Read the model definition and answer for the solid it produces. Units are mm, in the model's axes. A direction names the side the tool comes from. Round coordinates to 2 decimals unless told otherwise and drop trailing zeros. Loops run counter-clockwise (first coordinate to the right, second up) from the corner with the lowest first, then second, coordinate; pieces in that order, holes last. Notation, with made-up numbers: (31, 23.25) - (62, 23.25) arc R22 cw to (62, 57.25) - close; hole circle Ø7 at (-0.75, -3.75). An arc over 180 degrees is marked (long way). Use CSV: the item, a comma, the result in double quotes. Start each with the question number.
1. Consider line 1 along Y through (x, z) = (1.5, 0); line 2 along Z through (x, y) = (-34.5, -29); line 3 along X through (y, z) = (-25, 4). Determine where each line is inside the solid, lowest interval first.
2. A tool of negligible diameter and unlimited length cuts with its end or side. For faces 1 (the flat face through (1, -12.7, 7)), 2 (the flat face through (-19.164, -18, 5)), 3 (the flat face through (-12.7, -22.4, 9.3)), from which of +Z, -Z, +X, -X, +Y, -Y can it reach the whole face along a straight path? Write none if from no direction.
3. Find section D-D (z = 1.5). Give the vertices of the cut face in (x, y), and give its area (3 significant figures).
4. Given pin 1 Ø5.5 at (x, y) = (-29, -18.5) entering from +Z; pin 2 Ø5.5 at (x, z) = (-1.5, 10.5) entering from -Y; pin 3 Ø15 at (y, z) = (-27, 9) entering from +X, each flat-ended and moving along its own axis, determine where each tip first touches the part or whether it passes through.
5. Find section C-C (x = -9). Give the vertices of the cut face in (y, z).
6. Find section B-B (z = 13.5). Give the vertices of the cut face in (x, y).
7. Find section A-A (y = -8). Give the vertices of the cut face in (x, z), and give its area (3 significant figures).
from build123d import *

# Parameters (mm, degrees)
F0_W      = 50.8
F0_H      = 31.75
F1_DEPTH  = 31.75
F3_DEPTH  = 31.75
F5_DEPTH  = 19.05
F6_W      = 19.05
F6_H      = 18.953177
F7_DEPTH  = 19.05
F9_DEPTH  = 12.7
F11_DEPTH = 25.4


with BuildPart() as f1:
    # F0 (on Front) → F1 (new body)
    with BuildSketch(Plane.XZ):
        with Locations((-12.814426, 3.078177)):
            Rectangle(F0_W, F0_H)
    extrude(amount=F1_DEPTH)

    # F2 (on face) → F3 (cut)
    with BuildSketch(Plane.XZ.offset(31.75)):
        Polygon((12.585574, -0.096823), (12.585574, 18.953177), (0, 18.953177), align=None)
    extrude(amount=-F3_DEPTH, mode=Mode.SUBTRACT)

    # F4 (on face) → F5 (cut)
    with BuildSketch(Plane.XZ.offset(31.75)):
        Polygon((-6.35, 0), (12.585574, -0.096823), (0, 18.953177), (-6.35, 18.953177), align=None)
    extrude(amount=-F5_DEPTH, mode=Mode.SUBTRACT)

    # F6 (on face) → F7 (cut)
    with BuildSketch(Plane.XZ.offset(31.75)):
        with Locations((-28.689426, 9.476589)):
            Rectangle(F6_W, F6_H)
    extrude(amount=-F7_DEPTH, mode=Mode.SUBTRACT)

    # F8 (on face) → F9 (cut)
    with BuildSketch(Plane.YZ.offset(-6.35)):
        Polygon((-31.75, 0), (-12.7, 18.953177), (-31.75, 18.953177), align=None)
    extrude(amount=-F9_DEPTH, mode=Mode.SUBTRACT)

    # F10 (on face) → F11 (cut)
    with BuildSketch(Plane(origin=(-19.164426, 0, 0), x_dir=(0, -1, 0), z_dir=(-1, 0, 0))):
        Polygon((31.75, 18.953177), (12.7, 18.953177), (31.75, 0), align=None)
    extrude(amount=-F11_DEPTH, mode=Mode.SUBTRACT)


solid = f1.part
Filled sheet:
1,line 1,"y = -12.7 to 0"
1,line 2,"z = -12.8 to 0"
1,line 3,"x = -19.16 to -6.35"
2,face 1,"+Z, +X, -Y"
2,face 2,"+Z, -X, -Y"
2,face 3,"+Z, +X, -X, -Y"
3,outline,"(-38.21, -12.7) - (-19.16, -12.7) - (-19.16, -30.24) - (-6.35, -30.24) - (-6.35, -12.7) - (11.53, -12.7) - (11.53, 0) - (-38.21, 0) - close"
3,area,"857 mm²"
4,pin 1,"stops at z = 0"
4,pin 2,"stops at y = -12.7"
4,pin 3,"stops at x = -6.35"
5,outline,"(-31.75, -12.8) - (0, -12.8) - (0, 18.95) - (-12.7, 18.95) - (-31.75, 0) - close"
6,outline,"(-38.21, -12.7) - (-19.16, -12.7) - (-19.16, -18.18) - (-6.35, -18.18) - (-6.35, -12.7) - (3.6, -12.7) - (3.6, 0) - (-38.21, 0) - close"
7,outline,"(-38.21, -12.8) - (12.59, -12.8) - (12.59, -0.1) - (0, 18.95) - (-38.21, 18.95) - close"
7,area,"1,490 mm²"
